The listing builds one solid part. Answer for the finished solid, in the listing's coordinates (mm). Coordinates: 2 decimals unless noted, no trailing zeros. Loops run counter-clockwise (first coordinate to the right, second up) from the corner with the lowest first, then second, coordinate; pieces in that order, holes last. Notation, with made-up numbers: (-34, -18.5) - (23, -18.5) arc R14 ccw to (23, -5.5) - close; hole circle Ø9 at (12, -17). An arc over 180 degrees is marked (long way). Put each result on its own line as item: value.
```python
from build123d import *

# Parameters (mm, degrees)
F0_W     = 41
F0_H     = 90
F1_DEPTH = 34
F2_W     = 35
F2_H     = 29
F3_DEPTH = 86
F4_W     = 7
F4_H     = 6
F4_R     = 4
F4_R_2   = 1.55
F5_DEPTH = 4
F6_DEPTH = 86
F7_DEPTH = 2


with BuildPart() as f1:
    # F0 (on Top) → F1 (new body)
    with BuildSketch(Plane.XY):
        with Locations((-1.7023412511, 4.193077401)):
            Rectangle(F0_W, F0_H)
    extrude(amount=F1_DEPTH)

    # F2 (on face) → F3 (cut)
    with BuildSketch(Plane.XZ.offset(40.806922599)):
        with Locations((-1.7023412511, 17)):
            Rectangle(F2_W, F2_H)
    extrude(amount=-F3_DEPTH, mode=Mode.SUBTRACT)

    # F4 (on face) → F5 (cut, through all)
    with BuildSketch(Plane(origin=(0, 49.193077401, 0), x_dir=(-1, 0, 0), z_dir=(0, 1, 0))):
        with Locations((-10.2976587489, 7)):
            Rectangle(F4_W, F4_H)
        with Locations((1.7023412511, 17)):
            Circle(F4_R)
        with Locations((13.7023412511, 27)):
            Rectangle(F4_W, F4_H)
        with Locations((11.2023412511, 17)):
            Circle(F4_R_2)
        with Locations((-7.7976587489, 17)):
            Circle(F4_R_2)
        with Locations((1.7023412511, 25)):
            Circle(F4_R_2)
        with Locations((1.7023412511, 9)):
            Circle(F4_R_2)
    extrude(amount=-F5_DEPTH, mode=Mode.SUBTRACT)

    # F6 (cut): a face of the model
    f6_faces = [f1.faces().sort_by_distance(p)[0] for p in [
        (-21.6697062917, -40.806922599, 17),
    ]]
    extrude(f6_faces, amount=-F6_DEPTH, mode=Mode.SUBTRACT)

    # F7 (cut): a face of the model
    f7_faces = [f1.faces().sort_by_distance(p)[0] for p in [
        (-21.6697062917, 45.193077401, 17),
    ]]
    extrude(f7_faces, amount=-F7_DEPTH, mode=Mode.SUBTRACT)


solid = f1.part
```
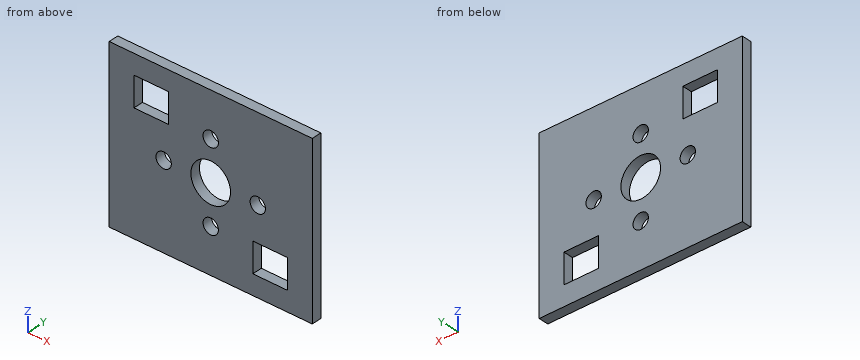
1) The part is cut by section B-B (x = -15). Give the vertices of the cut face in (y, z), and give its area (3 significant figures).
Found:
outline: (47.19, 0) - (49.19, 0) - (49.19, 24) - (47.19, 24) - close; (47.19, 30) - (49.19, 30) - (49.19, 34) - (47.19, 34) - close
area: 56.0 mm^2
2) The part is cut by section D-D (y = 48.7). Give the vertices of the cut face in (x, z), and give its area (3 significant figures).
Found:
outline: (-22.2, 0) - (18.8, 0) - (18.8, 34) - (-22.2, 34) - close; hole (-17.2, 24) - (-10.2, 24) - (-10.2, 30) - (-17.2, 30) - close; hole circle Ø3.1 at (-11.2, 17); hole circle Ø8 at (-1.7, 17); hole circle Ø3.1 at (-1.7, 9); hole circle Ø3.1 at (-1.7, 25); hole circle Ø3.1 at (7.8, 17); hole (6.8, 4) - (13.8, 4) - (13.8, 10) - (6.8, 10) - close
area: 1,230 mm^2
3) The part is cut by section C-C (z = 27.5). Give the vertices of the cut face in (x, y).
Found:
outline: (-22.2, 47.19) - (-17.2, 47.19) - (-17.2, 49.19) - (-22.2, 49.19) - close; (-10.2, 47.19) - (18.8, 47.19) - (18.8, 49.19) - (-10.2, 49.19) - close
4) The part is cut by section A-A (z = 17). Give the vertices of the cut face in (x, y).
Found:
outline: (-22.2, 47.19) - (-12.75, 47.19) - (-12.75, 49.19) - (-22.2, 49.19) - close; (-9.65, 47.19) - (-5.7, 47.19) - (-5.7, 49.19) - (-9.65, 49.19) - close; (2.3, 47.19) - (6.25, 47.19) - (6.25, 49.19) - (2.3, 49.19) - close; (9.35, 47.19) - (18.8, 47.19) - (18.8, 49.19) - (9.35, 49.19) - close
5) Straight lines are drawn through the part: L1, parallel to Z at x = 13, y = 47.4; L2, parallel to X at y = 48.8, z = 29; L3, parallel to Z at x = -3, y = 49.1. For each, find the intervals that lie inside material, in ascending order. Write a range as [from, to].
Found:
L1: z = [0, 4], [10, 34]
L2: x = [-22.2, -17.2], [-10.2, 18.8]
L3: z = [0, 8.15], [9.85, 13.22], [20.78, 24.15], [25.85, 34]
6) This flat-tipped pin is pushed along its axis until it touches: pin 1 (3 mm diameter, centred on x = -11.2, z = 17, fed in from -Y). Where does it stop, or does it pass through?
Found:
pin 1: passes through
